Verification items for the finished model (mm, model axes). Face numbers are marked on the shaded views. A direction names the side the tool comes from. Coordinates: 2 decimals unless noted, no trailing zeros. Order: outer loops, then holes, each group sorted by start corner. A loop starts at its lowest first (then second) coordinate and runs counter-clockwise, first axis right, second up. Notation, with made-up numbers: (-11, 32) -> (0, 32) arc R7 ccw to (0, 37) -> close; hole circle Ø10 at (54.25, 79). An arc over 180 degrees is marked (long way). Write item = value, one per line. Start each with the question number.
1. Cross-section at C-C on x = 0. Record the cut outline in (y, z), plus the area to 3 significant figures.
2. Cross-section at A-A on x = -22. Record the cut outline in (y, z).
3. Go/stop test with flat-tipped pins: P1, Ø5, axis at x = 14.5, y = -10, coming from the -Z side; P2, Ø10, axis at x = 18.5, y = 1.5, coming from the +Z side; P3, Ø4, axis at y = 2, z = 47, coming from the -X side; P4, Ø1.2, axis at y = 0, z = 106.5, coming from the -X side. Record where each tip stops, or that it passes through.
4. Set-up check for the marked faces 4, 5 and 6: record each of +Z, -Z, +X, -X, +Y, -Y from which the full face is reachable in a straight line by a thin tool's end or side.
5. Cross-section at D-D on y = -11.5. Record the cut outline in (x, z).
6. Cross-section at B-B on z = 102. Record the cut outline in (x, y), plus the area to 3 significant figures.
7. Release check for a two-part mould opening along Z. For the marked faces 1, 2 and 3 record: +Z half, -Z half, draft (parallel to the pull), parting line (faces both ways), or undercut.
8. Thickness scan on line 1 along Z through (x, y) = (-25, -3.5); line 2 along X through (y, z) = (-3, 103.5); line 3 along Z through (x, y) = (34.4, 0). Record the ranges inside material, lowest first. Write a range as from..to.
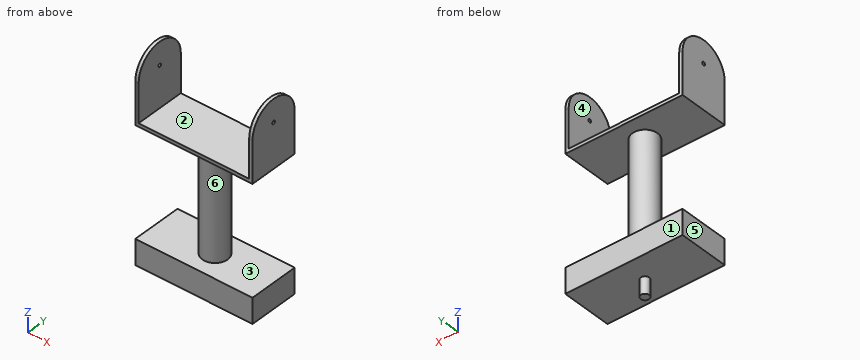
from build123d import *

# Parameters (mm, degrees)
F0_W      = 70
F0_H      = 30
F0_R      = 7.5
F0_R_2    = 2.5
F1_DEPTH  = 15
F2_DEPTH  = 10
F3_DEPTH  = 80
F4_W      = 66
F4_H      = 30
F4_R      = 7.5
F4_R_2    = 2.5
F4_W_2    = 2
F5_DEPTH  = 2
F6_DEPTH  = 25
F7_R      = 1
F8_DEPTH  = 2
F9_R      = 1
F10_DEPTH = 2


with BuildPart() as f1:
    # F0 (on Top) → F1 (new body)
    with BuildSketch(Plane.XY):
        Rectangle(F0_W, F0_H)
        Circle(F0_R, mode=Mode.SUBTRACT)
        Circle(F0_R)
        Circle(F0_R_2, mode=Mode.SUBTRACT)
        Circle(F0_R_2)
    extrude(amount=F1_DEPTH)

    # F0 (on Top) → F2 (join)
    with BuildSketch(Plane.XY):
        Circle(F0_R_2)
    extrude(amount=-F2_DEPTH)

    # F0 (on Top) → F3 (join)
    with BuildSketch(Plane.XY):
        Circle(F0_R)
        Circle(F0_R_2, mode=Mode.SUBTRACT)
    extrude(amount=F3_DEPTH)

    # F4 (on face) → F5 (join)
    with BuildSketch(Plane.XY.offset(80)):
        Rectangle(F4_W, F4_H)
        Circle(F4_R, mode=Mode.SUBTRACT)
        Circle(F4_R)
        Circle(F4_R_2, mode=Mode.SUBTRACT)
        Circle(F4_R_2)
        with Locations((-34, 0)):
            Rectangle(F4_W_2, F4_H)
        with Locations((34, 0)):
            Rectangle(F4_W_2, F4_H)
    extrude(amount=F5_DEPTH)

    # F4 (on face) → F6 (join)
    with BuildSketch(Plane.XY.offset(80)):
        with Locations((-34, 0)):
            Rectangle(F4_W_2, F4_H)
        with Locations((34, 0)):
            Rectangle(F4_W_2, F4_H)
    extrude(amount=F6_DEPTH)

    # F7 (on face) → F8 (join)
    with BuildSketch(Plane(origin=(-35, 0, 0), x_dir=(0, -1, 0), z_dir=(-1, 0, 0))):
        with BuildLine():
            Line((-15, 105), (15, 105))
            ThreePointArc((15, 105), (0, 120), (-15, 105))
        make_face()
        with Locations((0, 106.5)):
            Circle(F7_R, mode=Mode.SUBTRACT)
    extrude(amount=-F8_DEPTH)

    # F9 (on face) → F10 (join)
    with BuildSketch(Plane.YZ.offset(35)):
        with BuildLine():
            Line((-15, 105), (15, 105))
            ThreePointArc((15, 105), (0, 120), (-15, 105))
        make_face()
        with Locations((0, 106.5)):
            Circle(F9_R, mode=Mode.SUBTRACT)
    extrude(amount=-F10_DEPTH)


solid = f1.part
Worked out:
q1.outline = (-15, 0) -> (-2.5, 0) -> (-2.5, -10) -> (2.5, -10) -> (2.5, 0) -> (15, 0) -> (15, 15) -> (7.5, 15) -> (7.5, 80) -> (15, 80) -> (15, 82) -> (-15, 82) -> (-15, 80) -> (-7.5, 80) -> (-7.5, 15) -> (-15, 15) -> close; hole (-2.5, 15) -> (2.5, 15) -> (2.5, 80) -> (-2.5, 80) -> close
q1.area = 1,210 mm²
q2.outline = (-15, 0) -> (15, 0) -> (15, 15) -> (-15, 15) -> close; (-15, 80) -> (15, 80) -> (15, 82) -> (-15, 82) -> close
q3.P1 = 0
q3.P2 = 82
q3.P3 = -7.5
q3.P4 = through
q4.face_4 = +Z, +Y, -Y
q4.face_5 = +Z, -Z, -X, +Y, -Y
q4.face_6 = none
q5.outline = (-35, 0) -> (35, 0) -> (35, 15) -> (-35, 15) -> close; (-35, 80) -> (35, 80) -> (35, 114.63) -> (33, 114.63) -> (33, 82) -> (-33, 82) -> (-33, 114.63) -> (-35, 114.63) -> close
q6.outline = (-35, -15) -> (-33, -15) -> (-33, 15) -> (-35, 15) -> close; (33, -15) -> (35, -15) -> (35, 15) -> (33, 15) -> close
q6.area = 120 mm²
q7.face_1 = draft
q7.face_2 = +Z half
q7.face_3 = undercut
q8.line_1 = 0..15, 80..82
q8.line_2 = -35..-33, 33..35
q8.line_3 = 0..15, 80..105.5, 107.5..120
